Model file for the job. Use its own axes, mm. A direction names the side the tool comes from. Round coordinates to 2 decimals unless told otherwise and drop trailing zeros. Order: outer loops, then holes, each group sorted by start corner. A loop starts at its lowest first (then second) coordinate and runs counter-clockwise, first axis right, second up. Notation, with made-up numbers: M -22,46.5 L -15,46.5 A25 ccw -15,81.5 Z; hole C 41.5,10.25 d10. An arc over 180 degrees is marked long. Return JSON: item names as keys, results as strings. Group by question number.
Item 1: Slice it at B-B on y = 21.5. Write the cut outline in (x, z).
Item 2: Pull direction Z, two halves, no side cores. Call faces 1 (the face through (-33, 31, -3)), 2 (the face through (-34, 34, -1.016)), 3 (the face through (-16, 20, 0.984)), 4 (the face through (-16, 20, 33.984)): pulls with the +Z half, pulls with the -Z half, needs draft (parallel to the pull), parting line crosses it, or undercut.
Item 3: Slice it at D-D on x = -37. Write the cut outline in (y, z), then the cut area to 4 significant figures.
Item 4: Which spindle directions (+Z, -Z, +X, -X, +Y, -Y) get a long thin tool onto all of the face, cutting with end or side? Do faces 5 (the face through (-4.6, 5, -2)), 6 (the face through (-34.6, 20, 18)), 7 (the face through (-48.195, 1.014, 29.884)), 8 (the face through (-34, 10.8, -2)). Say none if no direction does.
Item 5: Slice it at A-A on x = -15.1. Write the cut outline in (y, z), then the cut area to 4 significant figures.
Item 6: Pin check, flat tips, straight feed: pin 1 Ø23.5 at (x, z) = (-52.1, 17.48) entering from -Y; pin 2 Ø8 at (x, z) = (-61, 3) entering from -Y; pin 3 Ø16.5 at (x, z) = (-45.5, 10.5) entering from +Y; pin 4 Ø1.2 at (x, z) = (-36.5, -3.5) entering from +Y. Stop position of each tip, or through.
Item 7: Slice it at C-C on z = 13.5. Write the cut outline in (x, y), then the cut area to 3 significant figures.
Item 8: Probe line 1 along X through (y, z) = (13, 6); line 2 along Z through (x, y) = (-44.5, 17.5); line 3 along Z through (x, y) = (-15, 1). List the from-to ranges inside material, lowest first.
from build123d import *

# Parameters (mm, degrees)
SKETCH1_W           = 74
SKETCH1_H           = 37
BOSS_EXTRUDE1_DEPTH = 37
SKETCH3_W           = 34
SKETCH3_H           = 33
CUT_EXTRUDE1_DEPTH  = 35
SKETCH5_R           = 13
CUT_EXTRUDE2_DEPTH  = 3.5
SKETCH6_W           = 74
SKETCH6_H           = 31
BOSS_EXTRUDE2_DEPTH = 4
CUT_EXTRUDE3_DEPTH  = 5.5


with BuildPart() as part:
    # Sketch1 → Boss-Extrude1 (new body)
    with BuildSketch(Plane(origin=(0, 0, 0), x_dir=(1, 0, 0), z_dir=(0, 1, 0))):
        with Locations((-33.6, -17.484146341)):
            Rectangle(SKETCH1_W, SKETCH1_H)
    extrude(amount=BOSS_EXTRUDE1_DEPTH)

    # Sketch3 → Cut-Extrude1 (cut)
    with BuildSketch(Plane(origin=(0, 37, 0), x_dir=(1, 0, 0), z_dir=(0, 1, 0))):
        with Locations((-51.6, -17.484146341)):
            Rectangle(SKETCH3_W, SKETCH3_H)
        with Locations((-15.6, -17.484146341)):
            Rectangle(SKETCH3_W, SKETCH3_H)
    extrude(amount=-CUT_EXTRUDE1_DEPTH, mode=Mode.SUBTRACT)

    # Sketch5 → Cut-Extrude2 (cut)
    with BuildSketch(Plane(origin=(0, 2, 0), x_dir=(1, 0, 0), z_dir=(0, 1, 0))):
        with Locations(Location((-15.1, -17.484146341, 0), (0, 0, 270))):
            Circle(SKETCH5_R)
        with Locations(Location((-52.1, -17.484146341, 0), (0, 0, 270))):
            Circle(SKETCH5_R)
    extrude(amount=-CUT_EXTRUDE2_DEPTH, mode=Mode.SUBTRACT)

    # Sketch6 → Boss-Extrude2 (add)
    with BuildSketch(Plane(origin=(0, 0, -1.015853659), x_dir=(-1, 0, 0), z_dir=(0, 0, -1))):
        with Locations((33.6, 15.5)):
            Rectangle(SKETCH6_W, SKETCH6_H)
    extrude(amount=BOSS_EXTRUDE2_DEPTH)

    # Sketch8 → Cut-Extrude3 (cut)
    with BuildSketch(Plane(origin=(0, 0, -5.015853659), x_dir=(-1, 0, 0), z_dir=(0, 0, -1))):
        Polygon((4.6, 29), (28.6, 29), (28.6, 13.8), (38.6, 13.8), (38.6, 29), (62.6, 29), (62.6, 13.8), (70.6, 13.8), (70.6, 10.8), (62.6, 10.8), (62.6, 0), (38.6, 0), (38.6, 10.8), (28.6, 10.8), (28.6, 0), (4.6, 0), (4.6, 10.8), (-3.4, 10.8), (-3.4, 13.8), (4.6, 13.8), align=None)
    extrude(amount=-CUT_EXTRUDE3_DEPTH, mode=Mode.SUBTRACT)


solid = part.part
Output values:
{
 "1": {"outline": "M -70.6,-5.02 L -62.6,-5.02 L -62.6,0.48 L -38.6,0.48 L -38.6,-5.02 L -28.6,-5.02 L -28.6,0.48 L -4.6,0.48 L -4.6,-5.02 L 3.4,-5.02 L 3.4,35.98 L -70.6,35.98 Z; hole M -68.6,0.98 L -34.6,0.98 L -34.6,33.98 L -68.6,33.98 Z; hole M -32.6,0.98 L 1.4,0.98 L 1.4,33.98 L -32.6,33.98 Z"},
 "2": {"face 1": "needs draft", "face 2": "pulls with the -Z half", "face 3": "undercut", "face 4": "undercut"},
 "3": {"outline": "M 0,-5.02 L 10.8,-5.02 L 10.8,0.48 L 13.8,0.48 L 13.8,-5.02 L 31,-5.02 L 31,-1.02 L 37,-1.02 L 37,0.98 L 2,0.98 L 2,33.98 L 37,33.98 L 37,35.98 L 0,35.98 Z", "area": "321.5 mm²"},
 "4": {"face 5": "-Z, -Y", "face 6": "+Y", "face 7": "+Y, -Y", "face 8": "-Z, +X, -X"},
 "5": {"outline": "M 0,0.48 L 29,0.48 L 29,-5.02 L 31,-5.02 L 31,-1.02 L 37,-1.02 L 37,0.98 L 2,0.98 L 2,4.48 L 0,4.48 Z; M 0,30.48 L 2,30.48 L 2,33.98 L 37,33.98 L 37,35.98 L 0,35.98 Z", "area": "126.5 mm²"},
 "6": {"pin 1": "through", "pin 2": "y = 0", "pin 3": "y = 2", "pin 4": "y = 31"},
 "7": {"outline": "M -70.6,0 L -64.47,0 L -64.47,2 L -68.6,2 L -68.6,37 L -70.6,37 Z; M -39.73,0 L -27.47,0 L -27.47,2 L -32.6,2 L -32.6,37 L -34.6,37 L -34.6,2 L -39.73,2 Z; M -2.73,0 L 3.4,0 L 3.4,37 L 1.4,37 L 1.4,2 L -2.73,2 Z", "area": "259 mm²"},
 "8": {"line 1": "-70.6 to -68.6, -34.6 to -32.6, 1.4 to 3.4", "line 2": "0.48 to 0.98, 33.98 to 35.98", "line 3": "0.48 to 4.48, 30.48 to 35.98"}
}
